The listing builds one solid part. Answer for the finished solid, in the listing's coordinates (mm). Face numbers are marked on the shaded views. Coordinates: 2 decimals unless noted, no trailing zeros. Write each loop counter-clockwise with the first axis right and the second up, starting at its lowest first coordinate (ties: lowest second). Pieces come first, ordered by that corner, then holes.
Autodesk Fusion 360 part; units mm, degrees
sketch "Sketch1" plane through (0, 0, 0) normal (1, 0, 0) x (0, 1, 0)
  circle A0 centre (0, 0) radius 45
  line L0 (-1.7761, 24.4773) -> (-1.7761, 15.686)
  line L1 (0.9712, 24.4773) -> (0.9712, 15.686)
  line L2 (-4.7479, 40.7242) -> (-4.7479, 37.8324)
  line L3 (-4.7479, 37.8324) -> (-1.6597, 37.8324)
  line L4 (-1.6597, 37.8324) -> (-1.6597, 34.0517)
  line L5 (-1.6597, 34.0517) -> (1.3885, 34.0517)
  line L6 (1.3885, 34.0517) -> (1.3885, 37.8324)
  line L7 (1.3885, 37.8324) -> (4.7125, 37.8324)
  line L8 (4.7125, 37.8324) -> (4.7125, 40.7283)
  line L9 (-6.6829, 7.2287) -> (-3.6696, 6.0858)
  line L10 (-3.6696, 6.0858) -> (-17.3847, -37.1318)
  line L11 (-17.7596, -36.954) -> (-16.1385, -25.606)
  line L12 (-16.1385, -25.606) -> (-6.6829, 7.2287)
  line L13 (0, 0) -> (0, -12.4098) construction
  line L14 (16.1385, -25.606) -> (6.6829, 7.2287)
  line L15 (3.6696, 6.0858) -> (17.3847, -37.1318)
  line L16 (6.6829, 7.2287) -> (3.6696, 6.0858)
  line L17 (17.7596, -36.954) -> (16.1385, -25.606)
  line L18 (15.1489, -14.4423) -> (17.5326, -21.9534)
  line L19 (19.4017, -21.3603) -> (16.9104, -13.7134)
  arc A1 (16.9561, -13.8536) -> (15.1489, -14.4423) centre (16.0297, -14.0779) ccw
  arc A2 (17.5326, -21.9534) -> (19.397, -21.346) centre (18.4671, -21.6568) ccw
  arc A3 (-9.6373, 17.866) -> (8.8324, 17.866) centre (-0.4024, 20.0816) ccw
  arc A4 (8.9914, 21.4775) -> (-9.7962, 21.4775) centre (-0.4024, 20.0816) ccw
  arc A5 (-12.0223, 17.866) -> (11.2175, 17.866) centre (-0.4024, 20.0816) ccw
  arc A6 (11.3442, 21.4775) -> (-12.149, 21.4775) centre (-0.4024, 20.0816) ccw
  line L20 (-12.149, 21.4775) -> (-9.7962, 21.4775)
  line L21 (-9.6373, 17.866) -> (-12.0223, 17.866)
  line L22 (11.2175, 17.866) -> (8.8324, 17.866)
  line L23 (8.9914, 21.4775) -> (11.3442, 21.4775)
  arc A7 (-1.7761, 24.4773) -> (-1.7761, 15.686) centre (-0.4024, 20.0816) ccw
  arc A8 (0.9712, 15.686) -> (0.9712, 24.4773) centre (-0.4024, 20.0816) ccw
  circle A9 centre (0, 0) radius 41
  dimension "d1" = 90
  dimension "d2" = 82
extrude "Extrude1" add sketch "Sketch1" along normal blind 10 contours A0 makes body 1
extrude "Extrude2" add sketch "Sketch1" along normal blind 6 contours L2 L3 L4 L5 L6 L7 L8 L9 L10 L11 L12 L14 L15 L16 L17 A9 bodies 1
fillet "Fillet1" radius 1.6 2 edges at (10, -38.2254, 14.8262) (10, -41.9547, -16.2727) on bodies 1
sketch "Sketch2" plane through (0, 0, 0) normal (1, 0, 0) x (0, 1, 0)
  line L0 (-68.9346, 55.3313) -> (70.9942, 55.3313)
  line L1 (70.9942, 55.3313) -> (70.9942, -61.2761)
  line L2 (70.9942, -61.2761) -> (-68.9346, -61.2761)
  line L3 (-68.9346, -61.2761) -> (-68.9346, 55.3313)
extrude "Extrude3" add sketch "Sketch2" along normal blind 14.803 separate body makes body 2
combine "Combine1" operation cut target body 2 tool bodies 1
fillet "Fillet2" radius 16.884 4 edges at (7.4015, 70.9942, -61.2761) (7.4015, 70.9942, 55.3313) (7.4015, -68.9346, -61.2761) (7.4015, -68.9346, 55.3313) on bodies 2
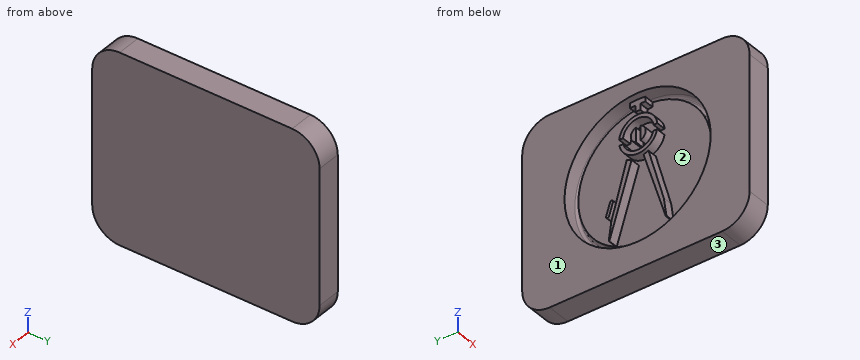
Q1. Find the intervals of material crossed by probe 1 along Z at (x, y) = (3, 0); probe 2 along Z at (x, y) = (7, 36.5); probe 3 along Y at (x, z) = (5, 13), in increasing order.
Answers below:
probe 1: z = -61.28 to -45, 8.26 to 10.59, 29.57 to 31.9, 34.05 to 41, 45 to 55.33
probe 2: z = -61.28 to -26.32, -18.67 to 18.67, 26.32 to 55.33
probe 3: y = -68.93 to -43.08, -9.88 to -6.73, 5.93 to 9.07, 43.08 to 70.99
Q2. Determine the mould class of the marked faces 1, 2 and 3 for opening direction Z: released by +Z, released by -Z, zero draft, split by the parting line, or undercut.
Answers below:
face 1: zero draft
face 2: undercut
face 3: released by -Z
Q3. Given pin 1 (6 mm diameter, centred on x = 7.5, y = 54.5, fed in from -Z), flat-ended and moving along its own axis, determine where the tip first touches the part or whether it passes through.
Answers below:
pin 1: stops at z = -61.28
Q4. The part is cut by section A-A, the plane x = 2. State how many separate pieces and enclosed holes the cut face has, then the cut area to 3 significant figures.
Answers below:
separate pieces: 9
enclosed holes: 1
area: 10,200 mm2
Q5. The part is cut by section B-B, the plane z = 0. Write down the section's boundary in (x, y), then the cut area to 3 significant figures.
Answers below:
outline: (0, -68.93) - (14.8, -68.93) - (14.8, 70.99) - (0, 70.99) - (0, 45) - (8.4, 45) arc R1.6 cw to (10, 43.4) - (10, 42.6) arc R1.6 cw to (8.4, 41) - (6, 41) - (6, 8.76) - (0, 8.76) - (0, 5.6) - (6, 5.6) - (6, -5.6) - (0, -5.6) - (0, -8.76) - (6, -8.76) - (6, -41) - (8.4, -41) arc R1.6 cw to (10, -42.6) - (10, -43.4) arc R1.6 cw to (8.4, -45) - (0, -45) - close
area: 1,540 mm2
